Verification items for the finished model (mm, model axes). A direction names the side the tool comes from. Round coordinates to 2 decimals unless told otherwise and drop trailing zeros. Order: outer loops, then holes, each group sorted by start corner. A loop starts at its lowest first (then second) coordinate and runs counter-clockwise, first axis right, second up. Notation, with made-up numbers: (63, 87.5) -> (112, 87.5) arc R10 ccw to (112, 93.5) -> close; hole circle Ø2 at (66.5, 62.5). An arc over 180 degrees is marked (long way). Return JSON: item names as keys, results as strings. Group by question number.
1) Draft check along Y on faces 5 (the flat face through (24, -5.105, 8)), 6 (the flat face through (0, -39.37, 49)), 7 (the flat face through (-26, 0, 38.1)). Enter one of: pulls with the +Y half, pulls with the -Y half, needs draft (parallel to the pull), parting line crosses it, or undercut.
2) Scan lines: L1, parallel to Y at x = -4.5, z = 12; L2, parallel to Y at x = -1.5, z = 53; L3, parallel to X at y = -18, z = 20.5. Record each from-to range of solid material in increasing order.
3) Section check D-D on y = 26.5. Enter the section's corners in (x, z).
4) Section check B-B on z = 32. Enter the section's corners in (x, y), plus the area to 3 significant figures.
5) Depth check by flat-ended pin: pin 1 (12 mm diameter, centred on x = -19, y = -22.5, fed in from -Z); pin 2 (3 mm diameter, centred on x = 24, y = -27, fed in from +Z); pin 3 (1 mm diameter, centred on y = 4.5, z = 7, fed in from +X); pin 4 (0.8 mm diameter, centred on x = 23.5, z = 10.5, fed in from +Y). Enter the tip coordinate at first touch or a pass-through.
6) Tool access check on faces 1 (the flat face through (24, -1, 15.455)), 2 (the flat face through (24, -31.369, 30)), 3 (the flat face through (0, -35.56, 21)), 4 (the flat face through (0, -36.83, 49)). Record the directions out of +Z, -Z, +X, -X, +Y, -Y that give a thin tool (end or side, any length) a straight path to the whole face; none if there is none.
7) Section check A-A on y = 10.5. Enter the section's corners in (x, z), plus the area to 3 significant figures.
8) Section check C-C on z = 13. Enter the section's corners in (x, y), plus the area to 3 significant figures.
```python
from build123d import *

# Parameters (mm, degrees)
F0_W          = 50.8
F0_H          = 38.1
F2_DEPTH      = 38.1
F2_DEPTH_BACK = 38.1
F3_DEPTH      = 39.37
F3_DEPTH_BACK = 39.37
F4_T          = -2.54
F6_W          = 9.1468244791
F6_H          = 15.4547751881
F6_W_2        = 8.080781489
F6_H_2        = 9.8759858869
F6_W_3        = 14.6728920285
F6_H_3        = 8.2574296976
F7_DEPTH      = 2.54


# Not quite as in the source:
# - the program builds the solid bodies; features that only make, move or delete a surface that nothing else refers to are left out


with BuildPart() as f2:
    # F0 (on Front) → F2 (new body, two sides)
    with BuildSketch(Plane.XZ) as f2_sk:
        with Locations((0, 19.05)):
            Rectangle(F0_W, F0_H)
    extrude(amount=F2_DEPTH)
    extrude(f2_sk.sketch, amount=-F2_DEPTH_BACK)

    # F1 (on Front) → F3 (join, two sides)
    with BuildSketch(Plane.XZ) as f3_sk:
        Polygon((0, 65.3146550722), (-26.7503901826, 38.1), (26.5896098174, 38.1), align=None)
    extrude(amount=F3_DEPTH)
    extrude(f3_sk.sketch, amount=-F3_DEPTH_BACK)

    # F4
    f4_openings = [f2.faces().sort_by_distance(p)[0] for p in [
        (0, 0, 0),
    ]]
    offset(amount=F4_T, openings=f4_openings, kind=Kind.INTERSECTION)

    # F6 (on offset) → F7 (cut)
    with BuildSketch(Plane.YZ.offset(25.4)):
        with Locations((-0.5318810698, 7.7273875941)):
            Rectangle(F6_W, F6_H)
        with Locations((-27.3286092555, 29.9121104646)):
            Rectangle(F6_W_2, F6_H_2)
        with Locations((-9.2311092555, 29.9121104646)):
            Rectangle(F6_W_2, F6_H_2)
        with Locations((8.8663907445, 29.9121104646)):
            Rectangle(F6_W_2, F6_H_2)
        with Locations((26.9638907445, 29.9121104646)):
            Rectangle(F6_W_2, F6_H_2)
        with Locations((24.2274460142, 11.3260603393)):
            Rectangle(F6_W_3, F6_H_3)
        with Locations((-24.0325539858, 11.3260603393)):
            Rectangle(F6_W_3, F6_H_3)
    extrude(amount=-F7_DEPTH, mode=Mode.SUBTRACT)


solid = f2.part
```
Check result:
{
 "1": {"face 5": "undercut", "face 6": "pulls with the -Y half", "face 7": "needs draft"},
 "2": {"L1": "-38.1 to -35.56, 35.56 to 38.1", "L2": "-39.37 to -36.83, 36.83 to 39.37", "L3": "-25.4 to -22.86, 22.86 to 25.4"},
 "3": {"outline": "(-26.75, 38.1) -> (-25.4, 38.1) -> (-25.4, 0) -> (-22.86, 0) -> (-22.86, 38.43) -> (-0.01, 61.69) -> (22.86, 38.28) -> (22.86, 34.85) -> (25.4, 34.85) -> (25.4, 38.1) -> (26.59, 38.1) -> (0, 65.31) -> close; (22.86, 0) -> (25.4, 0) -> (25.4, 7.2) -> (22.86, 7.2) -> close; (22.86, 15.45) -> (25.4, 15.45) -> (25.4, 24.97) -> (22.86, 24.97) -> close"},
 "4": {"outline": "(-25.4, -38.1) -> (25.4, -38.1) -> (25.4, -31.37) -> (22.86, -31.37) -> (22.86, -35.56) -> (-22.86, -35.56) -> (-22.86, 35.56) -> (22.86, 35.56) -> (22.86, 31) -> (25.4, 31) -> (25.4, 38.1) -> (-25.4, 38.1) -> close; (22.86, -23.29) -> (25.4, -23.29) -> (25.4, -13.27) -> (22.86, -13.27) -> close; (22.86, -5.19) -> (25.4, -5.19) -> (25.4, 4.83) -> (22.86, 4.83) -> close; (22.86, 12.91) -> (25.4, 12.91) -> (25.4, 22.92) -> (22.86, 22.92) -> close", "area": "537 mm^2"},
 "5": {"pin 1": "z = 0", "pin 2": "z = 42.29", "pin 3": "x = 25.4", "pin 4": "y = 38.1"},
 "6": {"face 1": "-Z, +X", "face 2": "+X", "face 3": "-Z", "face 4": "none"},
 "7": {"outline": "(-26.75, 38.1) -> (-25.4, 38.1) -> (-25.4, 0) -> (-22.86, 0) -> (-22.86, 38.43) -> (-0.01, 61.69) -> (22.86, 38.28) -> (22.86, 34.85) -> (25.4, 34.85) -> (25.4, 38.1) -> (26.59, 38.1) -> (0, 65.31) -> close; (22.86, 0) -> (25.4, 0) -> (25.4, 24.97) -> (22.86, 24.97) -> close", "area": "349 mm^2"},
 "8": {"outline": "(-25.4, -38.1) -> (25.4, -38.1) -> (25.4, -31.37) -> (22.86, -31.37) -> (22.86, -35.56) -> (-22.86, -35.56) -> (-22.86, 35.56) -> (22.86, 35.56) -> (22.86, 31.56) -> (25.4, 31.56) -> (25.4, 38.1) -> (-25.4, 38.1) -> close; (22.86, -16.7) -> (25.4, -16.7) -> (25.4, -5.11) -> (22.86, -5.11) -> close; (22.86, 4.04) -> (25.4, 4.04) -> (25.4, 16.89) -> (22.86, 16.89) -> close", "area": "522 mm^2"}
}
